```python
from build123d import *

# Parameters (mm, degrees)
BOSS_EXTRUDE1_DEPTH = 1.905
FILLET1_R           = 5.08
SKETCH2_W           = 12.7
SKETCH2_H           = 5.969
BOSS_EXTRUDE2_DEPTH = 1.905


with BuildPart() as part:
    # Sketch1 → Boss-Extrude1 (new body)
    with BuildSketch(Plane(origin=(0, 0, 0), x_dir=(1, 0, 0), z_dir=(0, 1, 0))):
        Polygon((19.05, 0), (31.75, 0), (31.75, 12.7), (-31.75, 12.7), (-31.75, 0), (-19.05, 0), (-19.05, -10.16), (-12.7, -10.16), (-12.7, -1.016), (12.7, -1.016), (12.7, -10.16), (19.05, -10.16), align=None)
    extrude(amount=BOSS_EXTRUDE1_DEPTH)

    # Fillet1
    fillet1_edges = [part.edges().sort_by_distance(p)[0] for p in [
        (-31.75, 0.9525, -12.7),
        (31.75, 0.9525, -12.7),
    ]]
    fillet(fillet1_edges, radius=FILLET1_R)

    # Sketch2 → Boss-Extrude2 (add)
    with BuildSketch(Plane(origin=(0, 1.905, 0), x_dir=(1, 0, 0), z_dir=(0, 1, 0))):
        with Locations((-12.7, -7.1755)):
            Rectangle(SKETCH2_W, SKETCH2_H)
        with Locations((12.7, -7.1755)):
            Rectangle(SKETCH2_W, SKETCH2_H)
    extrude(amount=-BOSS_EXTRUDE2_DEPTH)


solid = part.part
```
Can you work these out from the model? Positions are in its coordinate system, mm. A direction names the side the tool comes from. Round coordinates to 2 decimals unless told otherwise and drop trailing zeros. Order: outer loops, then holes, each group sorted by start corner. A loop starts at its lowest first (then second) coordinate and runs counter-clockwise, first axis right, second up.
(1) On a 3-axis mill with a long thin cutter (end or side, diameter ignored), from which of +Z, -Z, +X, -X, +Y, -Y can I reach the whole of each face in a straight line? I mean faces 1 (the face through (-31.75, 1, -4)), 2 (the face through (0, 1, 1.016)), 3 (the face through (-25, 1, 0)), 4 (the face through (19.05, 1, 5)), 5 (the face through (6.35, 1, 7)). Say none if no direction works.
Results are:
face 1: +Z, -Z, -X, +Y, -Y
face 2: +Y, -Y
face 3: +Z, -X, +Y, -Y
face 4: +Z, +X, +Y, -Y
face 5: +Z, +Y, -Y
(2) If we section it at A-A (x = -7.5): Please give me the cut outline in (y, z) (3 decimals), plus the area to 3 significant figures.
Results are:
outline: (0, -12.7) - (1.905, -12.7) - (1.905, 1.016) - (0, 1.016) - close; (0, 4.191) - (1.905, 4.191) - (1.905, 10.16) - (0, 10.16) - close
area: 37.5 mm2
(3) If I drill on L1, parallel to X at y = 0.15, z = 6; L2, parallel to Z at x = -23, y = 1.55; L3, parallel to Z at x = 3, y = 0.95, over which ranges is the centre line in solid material (lowest first)?
Results are:
L1: x = -19.05 to -6.35, 6.35 to 19.05
L2: z = -12.7 to 0
L3: z = -12.7 to 1.02
(4) We'd pull the mould along Z, two halves only. Please class faces 6 (the face through (9, 1, 4.191)), 7 (the face through (0, 1, -12.7)), 8 (the face through (-6.35, 1, 7)): +Z half, -Z half, draft (parallel to the pull), parting line (faces both ways), or undercut.
Results are:
face 6: undercut
face 7: -Z half
face 8: draft
(5) If we section it at D-D (x = -21): Please give me the cut outline in (y, z) (3 decimals).
Results are:
outline: (0, -12.7) - (1.905, -12.7) - (1.905, 0) - (0, 0) - close
(6) If we section it at B-B (z = 4.75): Please give me the cut outline in (x, y) (3 decimals).
Results are:
outline: (-19.05, 0) - (-6.35, 0) - (-6.35, 1.905) - (-19.05, 1.905) - close; (6.35, 0) - (19.05, 0) - (19.05, 1.905) - (6.35, 1.905) - close
(7) If we section it at C-C (y = 1.35): Please give me the cut outline in (x, z), plus the area to 3 significant figures.
Results are:
outline: (-31.75, -7.62) arc R5.08 ccw to (-26.67, -12.7) - (26.67, -12.7) arc R5.08 ccw to (31.75, -7.62) - (31.75, 0) - (19.05, 0) - (19.05, 10.16) - (6.35, 10.16) - (6.35, 4.19) - (12.7, 4.19) - (12.7, 1.02) - (-12.7, 1.02) - (-12.7, 4.19) - (-6.35, 4.19) - (-6.35, 10.16) - (-19.05, 10.16) - (-19.05, 0) - (-31.75, 0) - close
area: 1,030 mm2
(8) I'm going to push flat-ended pins straight in: pin 1 (1 mm diameter, centred on y = 1, z = 3.5, fed in from +X); pin 2 (0.6 mm diameter, centred on y = 1, z = 8, fed in from +X); pin 3 (1 mm diameter, centred on x = 25.5, y = 0.5, fed in from +Z). Where does each tip first touch, or does it pass through?
Results are:
pin 1: stops at x = 19.05
pin 2: stops at x = 19.05
pin 3: stops at z = 0
